The listing builds one solid part. Answer for the finished solid, in the listing's coordinates (mm). A direction names the side the tool comes from. Round coordinates to 2 decimals unless told otherwise and drop trailing zeros. Order: outer loops, then holes, each group sorted by start corner. A loop starts at its lowest first (then second) coordinate and runs counter-clockwise, first axis right, second up. Notation, with made-up numbers: M 44.25,-30.75 L 95.25,-30.75 A12 ccw 95.25,-14.75 Z; hole C -5,67.5 d7. An arc over 180 degrees is marked long. Write item = value, one per line. Start each with the question number.
(1) For a pull along Y with two mould halves and no side action, classify faces 4 (the face through (47, 241.3, 3)), 5 (the face through (3, 215.9, 3)), 6 (the face through (95.25, 82, 3)) as released by +Y, released by -Y, zero draft, split by the parting line, or undercut.
(2) Which of the six approach directions +Z, -Z, +X, -X, +Y, -Y give full straight-line access (tool end or side, diameter ignored) to faces 1 (the face through (92, 63.5, 3)), 2 (the face through (0, 235, 3)), 3 (the face through (3, 165.1, 3))?
(3) Each of these flat-tipped pins is pushed along its axis until it touches: pin 1 (2 mm diameter, centred on y = 194.5, z = 1, fed in from +X); pin 2 (3 mm diameter, centred on y = 43.5, z = 2.5, fed in from -X). Where does it stop, or does it pass through?
(4) A cutting plane is placed at A-A, the plane y = 144. Determine the outline of the cut face in (x, z).
(5) A straight line is drawn through the part: probe 1 along X at (y, z) = (222.5, 4.25). Find the intervals that lie inside material, in ascending order. Write a range as from..to.
from build123d import *

# Parameters (mm, degrees)
SKETCH1_W           = 95.25
SKETCH1_H           = 241.3
BOSS_EXTRUDE1_DEPTH = 6.35
SKETCH2_W           = 6.35
SKETCH2_H           = 12.7
CUT_EXTRUDE1_DEPTH  = 7.35
LPATTERN1_COUNT     = 9
LPATTERN1_PITCH     = 25.4


with BuildPart() as part:
    # Sketch1 → Boss-Extrude1 (new body)
    with BuildSketch(Plane.XY):
        with Locations((47.625, 120.65)):
            Rectangle(SKETCH1_W, SKETCH1_H)
    extrude(amount=BOSS_EXTRUDE1_DEPTH)

    # Sketch2 → Cut-Extrude1 (cut, through all)
    with BuildSketch(Plane.XY.offset(6.35)):
        with Locations((3.175, 222.25)):
            Rectangle(SKETCH2_W, SKETCH2_H)
        with Locations((92.075, 222.25)):
            Rectangle(SKETCH2_W, SKETCH2_H)
    cut_extrude1 = extrude(amount=-CUT_EXTRUDE1_DEPTH, mode=Mode.SUBTRACT)

    # LPattern1: Cut-Extrude1 ×9
    with Locations(*[(0, -i * LPATTERN1_PITCH, 0) for i in range(1, LPATTERN1_COUNT)]):
        add(cut_extrude1, mode=Mode.SUBTRACT)


solid = part.part
Reported:
q1.face_4 = released by +Y
q1.face_5 = undercut
q1.face_6 = zero draft
q2.face_1 = +Z, -Z, +X
q2.face_2 = +Z, -Z, -X, +Y, -Y
q2.face_3 = +Z, -Z, -X
q3.pin_1 = 88.9
q3.pin_2 = 6.35
q4.outline = M 6.35,0 L 88.9,0 L 88.9,6.35 L 6.35,6.35 Z
q5.probe_1 = 6.35..88.9
